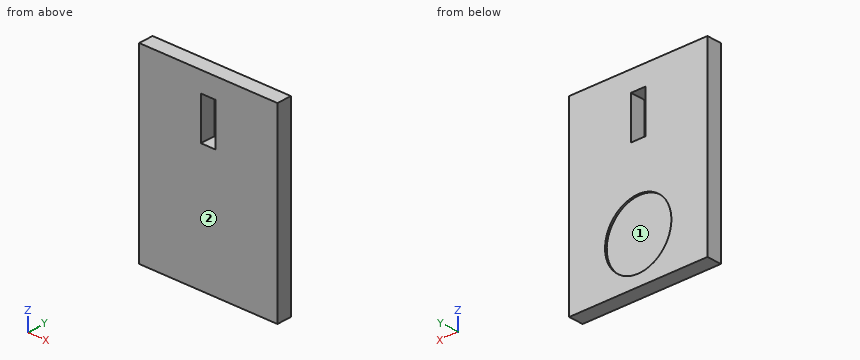
```python
from build123d import *

# Parameters (mm, degrees)
IZIM1_W                     = 150
IZIM1_H                     = 200
Y_KSEKLIK_EKSTR_ZYON1_DEPTH = 16
IZIM2_W                     = 16
IZIM2_H                     = 45
KES_EKSTR_ZYON1_DEPTH       = 29
IZIM3_R                     = 36
KES_EKSTR_ZYON3_DEPTH       = 2


with BuildPart() as part:
    # Çizim1 → Yükseklik-Ekstrüzyon1 (new body)
    with BuildSketch(Plane(origin=(0, 0, 0), x_dir=(1, 0, 0), z_dir=(0, 1, 0))):
        with Locations((-57.984293194, 82.460732984)):
            Rectangle(IZIM1_W, IZIM1_H)
    extrude(amount=Y_KSEKLIK_EKSTR_ZYON1_DEPTH)

    # Çizim2 → Kes-Ekstrüzyon1 (cut)
    with BuildSketch(Plane(origin=(0, 16, 0), x_dir=(1, 0, 0), z_dir=(0, 1, 0))):
        with Locations((-57.984293194, 26.373411694)):
            Rectangle(IZIM2_W, IZIM2_H)
    extrude(amount=-KES_EKSTR_ZYON1_DEPTH, mode=Mode.SUBTRACT)

    # Çizim3 → Kes-Ekstrüzyon3 (cut)
    with BuildSketch(Plane(origin=(0, 16, 0), x_dir=(1, 0, 0), z_dir=(0, 1, 0))):
        with Locations(Location((-57.984293194, 134.377130507, 0), (0, 0, 270))):
            Circle(IZIM3_R)
    extrude(amount=-KES_EKSTR_ZYON3_DEPTH, mode=Mode.SUBTRACT)


solid = part.part
```
Geometry: final body of the model. Coordinates: model frame, mm. Face numbers are marked on the shaded views. Round coordinates to 2 decimals unless told otherwise and drop trailing zeros. Order: outer loops, then holes, each group sorted by start corner. A loop starts at its lowest first (then second) coordinate and runs counter-clockwise, first axis right, second up. Notation, with made-up numbers: (-2.75, 4) - (29.25, 4) arc R14 ccw to (29.25, 14) - close; hole circle Ø7 at (31, -20). An arc over 180 degrees is marked (long way). Write item = value, one per line. Start each with the question number.
Q1. Ray query, line 1 (X direction, y = 11, z = -4); line 2 (Y direction, x = -89, z = -151); line 3 (Z direction, x = -53, y = 5). Return the intervals inside material, ascending. Write a range as from..to.
Q2. Cut plane B-B on y = 8.75. Return the cut outline in (x, z), and give its area (3 significant figures).
Q3. Pin query (flat end, axial travel): pin 1 (6 mm diameter, centred on x = -61, z = -109.5, fed in from +Y). Return the tip coordinate at first contact, or that it passes through.
Q4. Pull-direction query (X, two-part tool) for the marked faces 1 and 2; classes: +X half, -X half, draft (parallel to the pull), parting line (faces both ways), or undercut.
Q5. Cut plane A-A on x = -63. Return the cut outline in (y, z), and give its area (3 significant figures).
Q6. Cut plane C-C on z = -116.5. Return the cut outline in (x, y).
Q7. Cut plane D-D on x = -46.5. Return the cut outline in (y, z).
Outcome:
q1.line_1 = -132.98..-65.98, -49.98..17.02
q1.line_2 = 0..14
q1.line_3 = -182.46..-48.87, -3.87..17.54
q2.outline = (-132.98, -182.46) - (17.02, -182.46) - (17.02, 17.54) - (-132.98, 17.54) - close; hole (-65.98, -48.87) - (-49.98, -48.87) - (-49.98, -3.87) - (-65.98, -3.87) - close
q2.area = 29,300 mm^2
q3.pin_1 = 14
q4.face_1 = undercut
q4.face_2 = draft
q5.outline = (0, -182.46) - (16, -182.46) - (16, -170.03) - (14, -170.03) - (14, -98.73) - (16, -98.73) - (16, -48.87) - (0, -48.87) - close; (0, -3.87) - (16, -3.87) - (16, 17.54) - (0, 17.54) - close
q5.area = 2,340 mm^2
q6.outline = (-132.98, 0) - (17.02, 0) - (17.02, 16) - (-26.74, 16) - (-26.74, 14) - (-89.23, 14) - (-89.23, 16) - (-132.98, 16) - close
q7.outline = (0, -182.46) - (16, -182.46) - (16, -168.5) - (14, -168.5) - (14, -100.26) - (16, -100.26) - (16, 17.54) - (0, 17.54) - close
